Verification items for the finished model (mm, model axes). A direction names the side the tool comes from. Give positions to 0.01 mm unless a question says otherwise; leave off trailing zeros. Loops run counter-clockwise (first coordinate to the right, second up) from the corner with the lowest first, then second, coordinate; pieces in that order, holes last. Notation, with made-up numbers: (-35, 44) - (-14, 44) arc R14 cw to (-14, 63) - close; hole circle Ø10 at (-6, 37). An arc over 180 degrees is marked (long way). Put each result on its own line as item: value. Start each with the question number.
```python
from build123d import *

# Parameters (mm, degrees)
F1_DEPTH = 31.05
F2_W     = 58.1
F2_H     = 73.894663844
F3_DEPTH = 4


with BuildPart() as f1:
    # F0 (on Right) → F1 (new body, symmetric)
    with BuildSketch(Plane.YZ):
        with BuildLine():
            ThreePointArc((-35, 0), (-34.9856996834, 1.0004087475), (-34.9428104193, 2))
            Line((-34.9428104193, 2), (-37.947331922, 2))
            ThreePointArc((-37.947331922, 2), (-37.9868306985, 1.0003466807), (-38, 0))
            Line((-38, 0), (-35, 0))
        make_face()
        with BuildLine():
            ThreePointArc((-34.9428104193, 2), (0, 35), (34.9428104193, 2))
            Line((34.9428104193, 2), (37.947331922, 2))
            ThreePointArc((37.947331922, 2), (0, 38), (-37.947331922, 2))
            Line((-37.947331922, 2), (-34.9428104193, 2))
        make_face()
        with BuildLine():
            Line((1, 0), (35, 0))
            ThreePointArc((35, 0), (34.9856996834, 1.0004087475), (34.9428104193, 2))
            Line((34.9428104193, 2), (-34.9428104193, 2))
            ThreePointArc((-34.9428104193, 2), (-34.9856996834, 1.0004087475), (-35, 0))
            Line((-35, 0), (-1, 0))
            ThreePointArc((-1, 0), (0, 1), (1, 0))
        make_face()
        with BuildLine():
            ThreePointArc((34.9428104193, -2), (34.9856996834, -1.0004087475), (35, 0))
            Line((35, 0), (1, 0))
            ThreePointArc((1, 0), (0, -1), (-1, 0))
            Line((-1, 0), (-35, 0))
            ThreePointArc((-35, 0), (-34.9856996834, -1.0004087475), (-34.9428104193, -2))
            Line((-34.9428104193, -2), (34.9428104193, -2))
        make_face()
        with BuildLine():
            Line((-37.947331922, -2), (-34.9428104193, -2))
            ThreePointArc((-34.9428104193, -2), (-34.9856996834, -1.0004087475), (-35, 0))
            Line((-35, 0), (-38, 0))
            ThreePointArc((-38, 0), (-37.9868306985, -1.0003466807), (-37.947331922, -2))
        make_face()
        with BuildLine():
            Line((37.947331922, 0), (35, 0))
            ThreePointArc((35, 0), (34.9856996834, -1.0004087475), (34.9428104193, -2))
            Line((34.9428104193, -2), (37.947331922, -2))
            ThreePointArc((37.947331922, -2), (37.9868306985, -1.0003466807), (38, 0))
            Line((38, 0), (37.947331922, 0))
        make_face()
        with BuildLine():
            ThreePointArc((34.9428104193, 2), (34.9856996834, 1.0004087475), (35, 0))
            Line((35, 0), (37.947331922, 0))
            Line((37.947331922, 0), (37.947331922, 2))
            Line((37.947331922, 2), (34.9428104193, 2))
        make_face()
    extrude(amount=F1_DEPTH, both=True)

    # F2 (on face) → F3 (cut, through all)
    with BuildSketch(Plane(origin=(0, 0, -2), x_dir=(1, 0, 0), z_dir=(0, 0, -1))):
        Rectangle(F2_W, F2_H)
    extrude(amount=-F3_DEPTH, mode=Mode.SUBTRACT)


solid = f1.part
```
1) Set-up check for faces 1 (the face through (31.05, -3, 1.8)), 2 (the face through (-30, 0, 2)), 3 (the face through (0, 36, 2)): record each of +Z, -Z, +X, -X, +Y, -Y from which the full face is reachable in a straight line by a thin tool's end or side.
2) Draft check along Y on faces 4 (the face through (-29.05, 1, -1)), 5 (the face through (0.43, -1.17, 37.98)), 6 (the face through (0, 37.947, 1)). Enter one of: pulls with the +Y half, pulls with the -Y half, needs draft (parallel to the pull), parting line crosses it, or undercut.
3) Scan lines: line 1 along Y through (x, z) = (30.1, 0); line 2 along Y through (x, z) = (-9.5, 4); line 3 along Z through (x, y) = (16, 11.5). Record each from-to range of solid material in increasing order. Write a range as from..to.
4) Depth check by flat-ended pin: P1, Ø1, axis at x = -30.5, y = -7, coming from the +Z side; P2, Ø1, axis at x = 21.5, z = 4, coming from the +Y side; P3, Ø1.6, axis at x = 30.5, y = 17.5, coming from the +Z side. Enter the tip coordinate at first touch or a pass-through.
5) Section check C-C, the plane x = 26. Enter the section's corners in (y, z), plus the area to 3 significant figures.
6) Section check D-D, the plane y = -15. Enter the section's corners in (x, z), plus the area to 3 significant figures.
7) Section check B-B, the plane z = 4. Enter the section's corners in (x, y).
8) Section check A-A, the plane y = 0. Enter the section's corners in (x, z).
Results are:
1. face 1: +Z, -Z, +X, +Y, -Y
1. face 2: +X, -X
1. face 3: -Z
2. face 4: undercut
2. face 5: parting line crosses it
2. face 6: pulls with the +Y half
3. line 1: y = -38..-1, 1..37.95
3. line 2: y = -37.79..-34.77, 34.77..37.79
3. line 3: z = 33.06..36.22
4. P1: stops at z = 37.44
4. P2: stops at y = 37.84
4. P3: stops at z = 34.13
5. outline: (-37.95, -2) - (-36.95, -2) - (-36.95, 2) - (-34.94, 2) arc R35 cw to (34.94, 2) - (36.95, 2) - (36.95, -2) - (37.95, -2) arc R38 ccw to (38, 0) - (37.95, 0) - (37.95, 2) arc R38 ccw to start
5. area: 340 mm2
6. outline: (-31.05, -2) - (-29.05, -2) - (-29.05, 2) - (-31.05, 2) - close; (-31.05, 31.62) - (31.05, 31.62) - (31.05, 34.91) - (-31.05, 34.91) - close; (29.05, -2) - (31.05, -2) - (31.05, 2) - (29.05, 2) - close
6. area: 220 mm2
7. outline: (-31.05, -37.79) - (31.05, -37.79) - (31.05, -34.77) - (-31.05, -34.77) - close; (-31.05, 34.77) - (31.05, 34.77) - (31.05, 37.79) - (-31.05, 37.79) - close
8. outline: (-31.05, -2) - (-29.05, -2) - (-29.05, -1) - (-31.05, -1) - close; (-31.05, 1) - (-29.05, 1) - (-29.05, 2) - (-31.05, 2) - close; (-31.05, 35) - (31.05, 35) - (31.05, 38) - (-31.05, 38) - close; (29.05, -2) - (31.05, -2) - (31.05, -1) - (29.05, -1) - close; (29.05, 1) - (31.05, 1) - (31.05, 2) - (29.05, 2) - close
